Autodesk Inventor part; units mm, degrees
ref_plane "YZ Plane" through (0, 0, 0) normal (1, 0, 0) x (0, 1, 0)
ref_plane "XZ Plane" through (0, 0, 0) normal (0, 1, 0) x (-1, 0, 0)
ref_plane "XY Plane" through (0, 0, 0) normal (0, 0, 1) x (1, 0, 0)
sketch "Эскиз1" plane through (0, 0, 0) normal (0, 0, 1) x (1, 0, 0)
  ellipse E0 centre (0, 0) end of major axis (2.1776, -109.9784) minor radius 80 (68.6548, 55.2754) -> (68.6548, -57.6949) ccw
  circle A0 centre (0, 0) radius 17.5
  line L0 (-129.1764, 146.988) -> (-129.1764, 142.988) construction
  line L1 (-149.1764, 146.9879) -> (-129.1764, 146.988) construction
  line L2 (-149.1764, 142.9879) -> (-149.1764, 146.9879) construction
  line L3 (-129.1764, 142.988) -> (-149.1764, 142.9879) construction
  line L4 (-169.9145, 146.9879) -> (-169.9145, 142.9879) construction
  line L5 (-189.9145, 146.9878) -> (-169.9145, 146.9879) construction
  line L6 (-189.9145, 142.9878) -> (-189.9145, 146.9878) construction
  line L7 (-169.9145, 142.9879) -> (-189.9145, 142.9878) construction
  arc A1 (68.6548, 55.2754) -> (68.6548, -57.6949) centre (110, -1.2098) ccw
  line L8 (68.6548, 55.2754) -> (68.6548, -57.6949) construction
  line L9 (0, 109.9808) -> (0, -109.9808) construction
  line L10 (-2, -110) -> (2, -110)
  line L11 (2, -110) -> (2, -80)
  line L12 (2, -80) -> (-2, -80)
  line L13 (-2, -80) -> (-2, -110)
  line L14 (2, -110) -> (-2, -80) construction
  point P0 (0, -95)
  point P1 (0, -110)
  point P2 (-2, -109.9112)
  point P3 (2, -109.9817)
  dimension "d0" = 110
  dimension "d1" = 80
  dimension "d4" = 35
  dimension "d19" = 70
  dimension "d21" = 110
  dimension "d24" = 4
  dimension "d25" = 30
  dimension "d26" = 110
extrude "Выдавливание1" add sketch "Эскиз1" against normal blind 4 contours A1 E0 L11 L12 L13
fillet "Сопряжение1" radius 3 2 edges at (68.6548, 55.2754, -2) (68.6548, -57.6949, -2)
sketch "Эскиз5" plane through (0, 0, 0) normal (0, 0, 1) x (1, 0, 0)
  line L0 (-2, -110) -> (-2, -80)
  line L1 (-2, -80) -> (2, -80)
  line L2 (2, -80) -> (2, -110)
  line L3 (2, -110) -> (-2, -110)
  line L4 (-2, -34.6112) -> (2, -34.6112)
  line L5 (2, -64.6112) -> (-2, -64.6112)
  line L6 (-2, 65.3852) -> (2, 65.3852)
  line L7 (2, 35.3852) -> (-2, 35.3852)
  line L8 (-2, 80.7779) -> (-2, 110.7779)
  line L9 (-2, 110.7779) -> (2, 110.7779)
  line L10 (2, 110.7779) -> (2, 80.7779)
  line L11 (2, 80.7779) -> (-2, 80.7779)
  line L12 (-49.2252, -56.6111) -> (-46.452, -56.6111) construction
  line L13 (-46.452, -56.6111) -> (-46.452, -60.6111) construction
  line L14 (-46.452, -60.6111) -> (-49.2252, -60.6111) construction
  line L15 (-49.2252, -56.6111) -> (-49.2252, -60.6111) construction
  line L16 (-1.9986, -60.6111) -> (-31.9986, -60.6111)
  line L17 (-31.9986, -60.6111) -> (-31.9986, -56.6111)
  line L18 (-31.9986, -56.6111) -> (-1.9986, -56.6111)
  line L19 (2, -56.6111) -> (22.0269, -56.6111)
  line L20 (22.0269, -56.6111) -> (22.0269, -60.6111)
  line L21 (22.0269, -60.6111) -> (2, -60.6111)
  line L22 (42.765, -56.6111) -> (62.765, -56.6111)
  line L23 (62.765, -56.6111) -> (62.765, -60.6111)
  line L24 (62.765, -60.6111) -> (42.765, -60.6111)
  line L25 (42.765, -60.6111) -> (42.765, -56.6111)
  line L26 (-46.4535, 57.6183) -> (-49.2267, 57.6183) construction
  line L27 (-49.2267, 61.6183) -> (-49.2267, 57.6183) construction
  line L28 (-49.2267, 61.6183) -> (-46.4535, 61.6183) construction
  line L29 (-46.4535, 61.6183) -> (-46.4535, 57.6183) construction
  line L30 (-32.0001, 61.6183) -> (2, 61.6183)
  line L31 (-2.0001, 57.6186) -> (-2.0001, 57.6183)
  line L32 (2, 57.6183) -> (-32.0001, 57.6183)
  line L33 (-32.0001, 57.6183) -> (-32.0001, 61.6183)
  line L34 (62.7634, 61.6188) -> (62.7634, 57.6188)
  line L35 (42.7634, 61.6188) -> (62.7634, 61.6188)
  line L36 (62.7634, 57.6188) -> (42.7634, 57.6188)
  line L37 (42.7634, 57.6188) -> (42.7634, 61.6188)
  line L38 (22, 61.6187) -> (22, 57.6187)
  line L39 (22, 57.6187) -> (-2, 57.6186)
  line L40 (-2, 61.6186) -> (22, 61.6187)
  line L41 (-31.9986, -56.6111) -> (-46.452, -60.6111) construction
  circle A0 centre (-39.2253, -58.6111) radius 1.45
  line L42 (-2, -64.6112) -> (2, -80) construction
  circle A1 centre (0, -72.3056) radius 1.45
  line L43 (-46.4535, 57.6183) -> (-32.0001, 61.6183) construction
  circle A2 centre (-39.2268, 59.6183) radius 1.45
  line L44 (-2, 35.3852) -> (-2, 57.6186)
  line L45 (-2, 61.6183) -> (-2, 65.3852)
  line L46 (-2, -64.6112) -> (-2, -60.6111)
  line L47 (-2, -56.6111) -> (-2, -34.6112)
  line L48 (2, -34.6112) -> (2, -56.6111)
  line L49 (2, -60.6111) -> (2, -64.6112)
  line L50 (2, 65.3852) -> (2, 61.6186)
  line L51 (2, 57.6186) -> (2, 35.3852)
  line L52 (-2, 80.7779) -> (2, 65.3852) construction
  circle A3 centre (0, 73.0815) radius 1.45
  line L53 (2, 61.6186) -> (2, 57.6186)
  line L54 (-2, 57.6186) -> (-2, 61.6183)
  line L55 (2, -56.6111) -> (2, -60.6111)
  line L56 (-2, -60.6111) -> (-2, -56.6111)
  line L57 (42.7634, 61.6188) -> (22, 57.6187) construction
  circle A4 centre (32.3817, 59.6187) radius 1.45
  line L58 (42.765, -56.6111) -> (22.0269, -60.6111) construction
  circle A5 centre (32, -58.6874) radius 1.45
  point P0 (0, 0)
  point P1 (-2, 57.6183)
  dimension "d33" = 2.9
  dimension "d34" = 2.9
  dimension "d35" = 2.9
  dimension "d36" = 2.9
  dimension "d37" = 2.9
  dimension "d38" = 2.9
extrude "Выдавливание3" cut sketch "Эскиз5" against normal blind 4
sketch "Эскиз8" plane through (0, 0, 0) normal (0, 0, 1) x (1, 0, 0)
  circle A0 centre (14.8727, 14.8258) radius 1.55
  circle A1 centre (-14.8727, -14.8258) radius 1.55
  line L0 (0, 0) -> (0, 17.5) construction
  circle A2 centre (0, 0) radius 17.5 construction
  line L1 (-14.8727, -14.8258) -> (14.8727, -14.8258) construction
  line L2 (14.8727, -14.8258) -> (14.8727, 14.8258) construction
  line L3 (14.8727, 14.8258) -> (-14.8727, 14.8258) construction
  line L4 (-14.8727, 14.8258) -> (-14.8727, -14.8258) construction
  line L5 (-14.8727, -14.8258) -> (14.8727, 14.8258) construction
  circle A3 centre (-14.8727, 14.8258) radius 1.55
  circle A4 centre (14.8727, -14.8258) radius 1.55
  dimension "d39" = 3.1
  dimension "d40" = 3.1
  dimension "d46" = 3.1
  dimension "d47" = 3.1
extrude "Выдавливание6" cut sketch "Эскиз8" against normal blind 10
properties part number "верхний эллипс туловища"
Check sheet for the modelled part. Datum: model origin and axes. Units: mm. A direction names the side the tool comes from. Round coordinates to 2 decimals unless told otherwise and drop trailing zeros. Answer as a JSON object with one key per item and string values. Group by question number.
Q1. Sectioned sample at A-A, the plane x = 47. Count the separate pieces of the cut face and the enclosed holes in it, plus the area to 3 significant figures.
Q2. Mould release check, pull along X, two halves, no side actions. Record for faces 5 (the face through (40.006, -0.315, -1.972)), 6 (the face through (12, -56.611, -2)), 7 (the face through (-17, -60.611, -2)), 8 (the face through (-24, 2, -4)): released by +X, released by -X, zero draft, split by the parting line, or undercut.
Q3. Scan lines: line 1 along Y through (x, z) = (-24.5, -2.25); line 2 along Y through (x, z) = (0.5, -2.85); line 3 along Y through (x, z) = (-6.5, -1.1). Record each from-to range of solid material in increasing order. Write a range as [from, to].
Q4. Set-up check for faces 1 (the face through (-24, 2, 0)), 2 (the face through (53, 57.619, -2)), 3 (the face through (2, 96, -2)), 4 (the face through (-2, -95, -2)): record each of +Z, -Z, +X, -X, +Y, -Y from which the full face is reachable in a straight line by a thin tool's end or side.
Q5. Gauge pin test, flat ends, axial feed: P1, Ø1.5, axis at x = -55, z = -3, coming from the -Y side; P2, Ø2, axis at y = 32.5, z = -1, coming from the +X side; P3, Ø2, axis at x = -14.5, z = -2, coming from the +Y side. Record the tip position at first contact, or that the pin passes through.
Solution:
{
 "1": {"separate pieces": "4", "enclosed holes": "0", "area": "436 mm²"},
 "2": {"face 5": "released by +X", "face 6": "undercut", "face 7": "undercut", "face 8": "zero draft"},
 "3": {"line 1": "y = [-104.27, -60.61], [-56.61, 57.62], [61.62, 105.13]", "line 2": "y = [-80, -73.67], [-70.94, -64.61], [-34.61, -17.49], [17.49, 35.39], [65.39, 71.72], [74.44, 80.78]", "line 3": "y = [-109.5, -60.61], [-56.61, -16.25], [16.25, 57.62], [61.62, 109.73]"},
 "4": {"face 1": "+Z, +X, -X, +Y, -Y", "face 2": "+Z, -Z", "face 3": "+Z, -Z, +Y", "face 4": "+Z, -Z, -Y"},
 "5": {"P1": "stops at y = -79.89", "P2": "stops at x = 49.21", "P3": "stops at y = 108.64"}
}
